The drawing under review shows one solid part. Ordinate dimensions are in mm from its lowest x, y, z. A direction names the side the tool comes from. Round coordinates to 2 decimals unless told otherwise and drop trailing zeros. Write each loop counter-clockwise with the first axis right and the second up, starting at its lowest first coordinate (ties: lowest second). Pieces come first, ordered by that corner, then holes. Notation, with made-up numbers: M 77.25,63 L 134.25,63 A9 cw 134.25,77 Z; hole C 47,24.25 d9. An arc over 180 degrees is marked long. Write item = value, one per line. Start each with the question number.
Item 1: Take a section at C-C, the plane x = 88. Give the boundary of the cut face in (y, z).
Item 2: Take a section at B-B, the plane y = 79.5. Give the boundary of the cut face in (x, z) (1 decimal).
Item 3: To check wall thickness, follow line 1 along Z through (x, y) = (79, 81); line 2 along Y through (x, z) = (51.5, 20.5); line 3 along Y through (x, z) = (97, 37) (1 decimal). State the ranges of each line that lie inside material, in increasing order.
Item 4: Tool access review of the marked faces 4 and 5: name each direction out of +Z, -Z, +X, -X, +Y, -Y from which nothing blocks a thin tool from reaching the whole face with its end or side.
Item 5: Take a section at A-A, the plane z = 11. Give the boundary of the cut face in (x, y) (1 decimal), plus the area to 3 significant figures.
Item 6: The part is to be moulded in two halves that separate along X. For the marked faces 1, 2 and 3, say which applies: +X half, -X half, draft (parallel to the pull), parting line (faces both ways), or undercut.
Item 7: For pin 1 Ø3 at (x, y) = (79.5, 83.5) entering from +Z; pin 2 Ø10 at (x, z) = (73.5, 23) entering from -Y; pin 3 Ø2 at (y, z) = (15.5, 30.5) entering from +X; pin 4 Ø1.5 at (y, z) = (27.5, 12.5) entering from -X, all flat-tipped, find the tip position at first contact; note any pin that passes through.
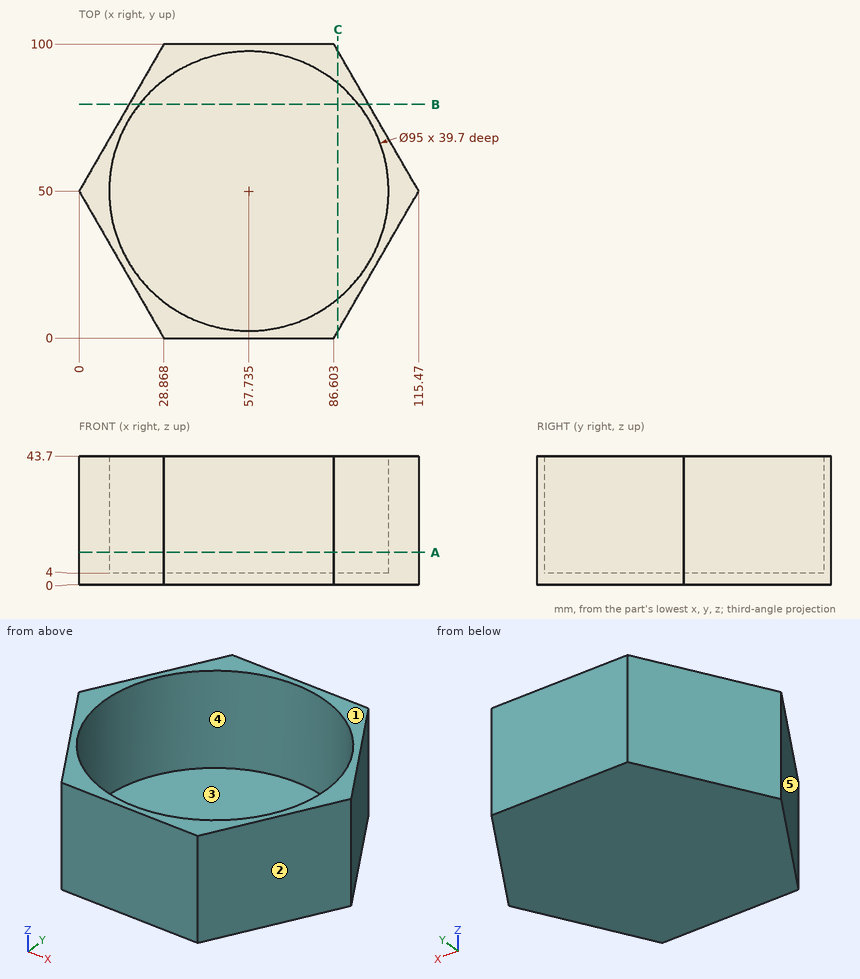
Response values:
q1.outline = M 2.42,0 L 97.58,0 L 97.58,43.7 L 86.61,43.7 L 86.61,4 L 13.39,4 L 13.39,43.7 L 2.42,43.7 Z
q2.outline = M 17,0 L 98.4,0 L 98.4,43.7 L 95,43.7 L 95,4 L 20.5,4 L 20.5,43.7 L 17,43.7 Z
q3.line_1 = 0 to 4
q3.line_2 = 0 to 2.91, 97.09 to 100
q3.line_3 = 18 to 23.3, 76.7 to 82
q4.face_4 = +Z
q4.face_5 = +Z, -Z, -X, -Y
q5.outline = M 0,50 L 28.9,0 L 86.6,0 L 115.5,50 L 86.6,100 L 28.9,100 Z; hole C 57.7,50 d95
q5.area = 1,570 mm2
q6.face_1 = draft
q6.face_2 = +X half
q6.face_3 = undercut
q7.pin_1 = 4
q7.pin_2 = 0
q7.pin_3 = 96.13
q7.pin_4 = 12.56
